```python
from build123d import *

# Parameters (mm, degrees)
F0_R      = 9.525
F1_DEPTH  = 25.4
F1_FACE_R = 9.525
F2_DEPTH  = 25.4
F4_DEPTH  = 50.801
F6_DEPTH  = 9.525
F7_W      = 11.0998
F7_H      = 11.0998
F8_DEPTH  = 12.7


with BuildPart() as f1:
    # F0 (on Front) → F1 (new body)
    with BuildSketch(Plane.XZ):
        Circle(F0_R)
    extrude(amount=F1_DEPTH)

    # F1_face (on face) → F2 (join)
    with BuildSketch(Plane.XZ.offset(25.4)):
        Circle(F1_FACE_R)
    extrude(amount=F2_DEPTH)

    # F3 (on Front) → F4 (cut, through all)
    with BuildSketch(Plane.XZ):
        with BuildLine():
            ThreePointArc((4.7625, 0), (3.367596, 3.367596), (0, 4.7625))
            ThreePointArc((0, 4.7625), (-3.367596, 3.367596), (-4.7625, 0))
            ThreePointArc((-4.7625, 0), (-3.367596, -3.367596), (0, -4.7625))
            ThreePointArc((0, -4.7625), (3.367596, -3.367596), (4.7625, 0))
        make_face()
    extrude(amount=F4_DEPTH, mode=Mode.SUBTRACT)

    # F5 (on face) → F6 (cut)
    with BuildSketch(Plane(origin=(0, 0, 0), x_dir=(-1, 0, 0), z_dir=(0, 1, 0))):
        Polygon((3.65125, 6.324151), (-3.65125, 6.324151), (-7.3025, 0), (-3.65125, -6.324151), (3.65125, -6.324151), (7.3025, 0), align=None)
    extrude(amount=-F6_DEPTH, mode=Mode.SUBTRACT)

    # F7 (on face) → F8 (cut)
    with BuildSketch(Plane.XZ.offset(50.8)):
        Rectangle(F7_W, F7_H)
    extrude(amount=-F8_DEPTH, mode=Mode.SUBTRACT)


solid = f1.part
```
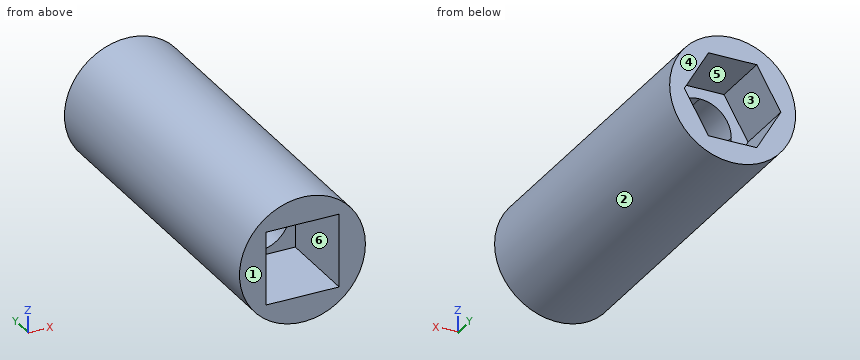
Here's how the part is built. I have some questions about the finished solid (model axes, mm). Face numbers are marked on the shaded views. A direction names the side the tool comes from. Coordinates: 2 decimals unless noted, no trailing zeros. Order: outer loops, then holes, each group sorted by start corner. A loop starts at its lowest first (then second) coordinate and runs counter-clockwise, first axis right, second up. Notation, with made-up numbers: (-7.5, 17.25) -> (14.5, 17.25) arc R17 ccw to (14.5, 33.25) -> close; hole circle Ø4 at (-16, 81.5). An arc over 180 degrees is marked (long way). Return JSON: item names as keys, results as strings.
1) Thinking about a two-plate mould opening in Z: for the marked faces 1, 2 and 3, which applies, +Z half, -Z half, draft (parallel to the pull), parting line (faces both ways), or undercut?
Conclusion:
{"face 1": "draft", "face 2": "parting line", "face 3": "undercut"}
2) If we section it at C-C on z = -3.5: List the corners of the cut face in (x, y) for me (3 decimals).
Conclusion:
{"outline": "(-8.859, -50.8) -> (-5.55, -50.8) -> (-5.55, -38.1) -> (-3.23, -38.1) -> (-3.23, -9.525) -> (-5.282, -9.525) -> (-5.282, 0) -> (-8.859, 0) -> close; (3.23, -38.1) -> (5.55, -38.1) -> (5.55, -50.8) -> (8.859, -50.8) -> (8.859, 0) -> (5.282, 0) -> (5.282, -9.525) -> (3.23, -9.525) -> close"}
3) On a 3-axis mill with a long thin cutter (end or side, diameter ignored), from which of +Z, -Z, +X, -X, +Y, -Y can I reach the whole of each face in a straight line? I mean the marked faces 4, 5 and 6. Say none if no direction works.
Conclusion:
{"face 4": "+Z, -Z, +X, -X, +Y", "face 5": "+Y", "face 6": "-Y"}
4) I'm going to push flat-ended pins straight in: P1, Ø3.5, axis at y = -44.5, z = -3, coming from the +X side; P2, Ø6, axis at x = -7, y = -15.5, coming from the +Z side; P3, Ø2, axis at x = 1, z = 5, coming from the +Y side (3 decimals). Where does each tip first touch, or does it pass through?
Conclusion:
{"P1": "stops at x = 9.44", "P2": "stops at z = 8.64", "P3": "stops at y = -9.525"}
5) If I drill on probe 1 along Y at (x, z) = (-2.25, 5.5) (3 decimals); probe 2 along X at (y, z) = (-4, 1.5); probe 3 along X at (y, z) = (-38.5, 4.75), over which ranges is the centre line in solid material (lowest first)?
Conclusion:
{"probe 1": "y = -38.1 to -9.525", "probe 2": "x = -9.41 to -6.44, 6.44 to 9.41", "probe 3": "x = -8.26 to -5.55, 5.55 to 8.26"}
6) If we section it at B-B on y = -45: List the corners of the cut face in (x, z) for me (3 decimals), plus the area to 3 significant figures.
Conclusion:
{"outline": "circle Ø19.05 at (0, 0); hole (-5.55, -5.55) -> (5.55, -5.55) -> (5.55, 5.55) -> (-5.55, 5.55) -> close", "area": "162 mm²"}
7) If we section it at A-A on x = -0.5: List the corners of the cut face in (y, z) for me (3 decimals).
Conclusion:
{"outline": "(-50.8, -9.512) -> (0, -9.512) -> (0, -6.324) -> (-9.525, -6.324) -> (-9.525, -4.736) -> (-38.1, -4.736) -> (-38.1, -5.55) -> (-50.8, -5.55) -> close; (-50.8, 5.55) -> (-38.1, 5.55) -> (-38.1, 4.736) -> (-9.525, 4.736) -> (-9.525, 6.324) -> (0, 6.324) -> (0, 9.512) -> (-50.8, 9.512) -> close"}
